Can you work these out from the model? Positions are in its coordinate system, mm. Face numbers are marked on the shaded views. A direction names the side the tool comes from. Give positions to 0.01 mm unless a question says otherwise; leave off trailing zeros. Loops run counter-clockwise (first coordinate to the right, second up) from the corner with the lowest first, then second, coordinate; pieces in that order, holes last. Notation, with made-up numbers: (46.25, 84.5) -> (74.25, 84.5) arc R31 cw to (74.25, 111.5) -> close; hole circle Ø7 at (50.25, -3.75). An arc over 180 degrees is marked (long way). Return JSON: item names as keys, results as strings. Group by question number.
Q1. Suppose I cut it at B-B, the plane z = 5. Please give me the cut outline in (x, y), and give its area (3 significant figures).
Q2. Thinking about a two-plate mould opening in Z: for the marked faces 1, 2, 3 and 4, which applies, pulls with the +Z half, pulls with the -Z half, needs draft (parallel to the pull), parting line crosses it, or undercut?
Q3. Suppose I cut it at D-D, the plane x = -15.5. Please give me the cut outline in (y, z).
Q4. Which directions (+Z, -Z, +X, -X, +Y, -Y) give clear straight access to the entire face, cutting with the end or side of a thin tool? Please do the marked faces 5 and 6.
Q5. Will these pins go through, and if not, where does the flat tip stop? pin 1 (5.5 mm diameter, centred on y = 0, z = 0, fed in from +X); pin 2 (5 mm diameter, centred on y = 2.5, z = -17, fed in from -X); pin 3 (4 mm diameter, centred on y = 5, z = -5, fed in from -X).
Q6. Suppose I cut it at C-C, the plane z = -2. Please give me the cut outline in (x, y).
Q7. I need wall thicknesses on line 1 along Y through (x, z) = (-15.5, 20.95); line 2 along Y through (x, z) = (-8, -21.35); line 3 along Y through (x, z) = (17.25, 5). Which ranges of each line are inside material? Lowest first, please. Write a range as [from, to].
Q8. Suppose I cut it at A-A, the plane x = 10. Please give me the cut outline in (y, z), and give its area (3 significant figures).
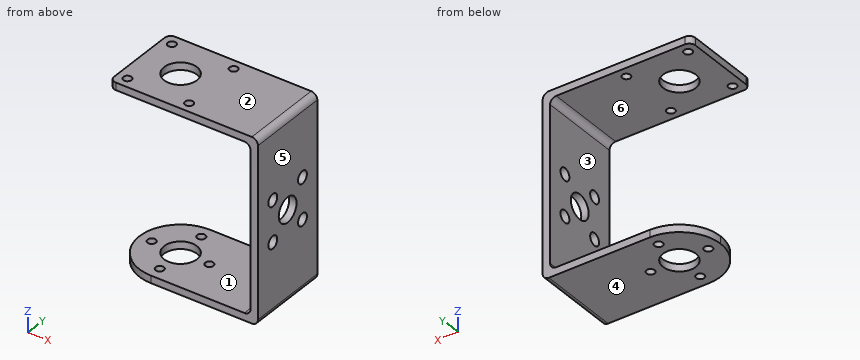
```python
from build123d import *

# Parameters (mm, degrees)
BOSS_EXTRUDE1_DEPTH = 10
FILLET1_R           = 1.5
CUT_EXTRUDE1_DEPTH  = 2
SKETCH4_R           = 4
CUT_EXTRUDE3_DEPTH  = 45.2
SKETCH6_R           = 3
SKETCH6_R_2         = 1.5
CUT_EXTRUDE4_DEPTH  = 2
SKETCH7_R           = 1
CUT_EXTRUDE5_DEPTH  = 2
SKETCH8_R           = 1
CUT_EXTRUDE6_DEPTH  = 2


with BuildPart() as part:
    # Sketch1 → Boss-Extrude1 (new body, symmetric)
    with BuildSketch(Plane(origin=(0, 0, 0), x_dir=(1, 0, 0), z_dir=(0, 1, 0))):
        Polygon((-18, 20.3), (16.2, 20.3), (16.2, -20.3), (-18, -20.3), (-18, -22.1), (18, -22.1), (18, 22.1), (-18, 22.1), align=None)
    extrude(amount=BOSS_EXTRUDE1_DEPTH, both=True)

    # Fillet1
    fillet1_edges = [part.edges().sort_by_distance(p)[0] for p in [
        (18, 0, -22.1),
        (18, 0, 22.1),
        (16.2, 0, 20.3),
        (16.2, 0, -20.3),
        (-18, 10, 21.2),
        (-18, -10, 21.2),
    ]]
    fillet(fillet1_edges, radius=FILLET1_R)

    # Sketch2 → Cut-Extrude1 (cut)
    with BuildSketch(Plane(origin=(0, 0, -22.1), x_dir=(-1, 0, 0), z_dir=(0, 0, -1))):
        with BuildLine():
            Line((18, 10), (8, 10))
            ThreePointArc((8, 10), (15.071067812, 7.071067812), (18, 0))
            Line((18, 0), (18, 10))
        make_face()
        with BuildLine():
            Line((18, -10), (18, 0))
            ThreePointArc((18, 0), (15.071067812, -7.071067812), (8, -10))
            Line((8, -10), (18, -10))
        make_face()
    extrude(amount=-CUT_EXTRUDE1_DEPTH, mode=Mode.SUBTRACT)

    # Sketch4 → Cut-Extrude3 (cut, through all)
    with BuildSketch(Plane.XY.offset(22.1)):
        with Locations((-8, 0)):
            Circle(SKETCH4_R)
    extrude(amount=-CUT_EXTRUDE3_DEPTH, mode=Mode.SUBTRACT)

    # Sketch6 → Cut-Extrude4 (cut)
    with BuildSketch(Plane.ZY.offset(-16.2)):
        Circle(SKETCH6_R)
        with Locations((5, -5)):
            Circle(SKETCH6_R_2)
        with Locations((-5, -5)):
            Circle(SKETCH6_R_2)
        with Locations((-5, 5)):
            Circle(SKETCH6_R_2)
        with Locations((5, 5)):
            Circle(SKETCH6_R_2)
    extrude(amount=-CUT_EXTRUDE4_DEPTH, mode=Mode.SUBTRACT)

    # Sketch7 → Cut-Extrude5 (cut)
    with BuildSketch(Plane.XY.offset(22.1)):
        with Locations((-15.5, -7.5)):
            Circle(SKETCH7_R)
        with Locations((-15.5, 7.5)):
            Circle(SKETCH7_R)
        with Locations((-0.5, 7.5)):
            Circle(SKETCH7_R)
        with Locations((-0.5, -7.5)):
            Circle(SKETCH7_R)
    extrude(amount=-CUT_EXTRUDE5_DEPTH, mode=Mode.SUBTRACT)

    # Sketch8 → Cut-Extrude6 (cut)
    with BuildSketch(Plane(origin=(0, 0, -22.1), x_dir=(-1, 0, 0), z_dir=(0, 0, -1))):
        with Locations((8, -7)):
            Circle(SKETCH8_R)
        with Locations((15, 0)):
            Circle(SKETCH8_R)
        with Locations((8, 7)):
            Circle(SKETCH8_R)
        with Locations((1, 0)):
            Circle(SKETCH8_R)
    extrude(amount=-CUT_EXTRUDE6_DEPTH, mode=Mode.SUBTRACT)


solid = part.part
```
Ans:
{
 "1": {"outline": "(16.2, -10) -> (18, -10) -> (18, -6.5) -> (16.2, -6.5) -> close; (16.2, -3.5) -> (18, -3.5) -> (18, 3.5) -> (16.2, 3.5) -> close; (16.2, 6.5) -> (18, 6.5) -> (18, 10) -> (16.2, 10) -> close", "area": "25.2 mm^2"},
 "2": {"face 1": "undercut", "face 2": "pulls with the +Z half", "face 3": "undercut", "face 4": "pulls with the -Z half"},
 "3": {"outline": "(-10, 20.3) -> (-8.5, 20.3) -> (-8.5, 22.1) -> (-10, 22.1) -> close; (-6.61, -22.1) -> (-0.87, -22.1) -> (-0.87, -20.3) -> (-6.61, -20.3) -> close; (-6.5, 20.3) -> (6.5, 20.3) -> (6.5, 22.1) -> (-6.5, 22.1) -> close; (0.87, -22.1) -> (6.61, -22.1) -> (6.61, -20.3) -> (0.87, -20.3) -> close; (8.5, 20.3) -> (10, 20.3) -> (10, 22.1) -> (8.5, 22.1) -> close"},
 "4": {"face 5": "+Z, -Z, +X, +Y, -Y", "face 6": "-X, +Y, -Y"},
 "5": {"pin 1": "passes through", "pin 2": "stops at x = 16.03", "pin 3": "stops at x = 16.2"},
 "6": {"outline": "(16.2, -10) -> (18, -10) -> (18, -2.24) -> (16.2, -2.24) -> close; (16.2, 2.24) -> (18, 2.24) -> (18, 10) -> (16.2, 10) -> close"},
 "7": {"line 1": "y = [-10, -8.5], [-6.5, 6.5], [8.5, 10]", "line 2": "y = [-10, -8], [-6, -4], [4, 6], [8, 10]", "line 3": "y = [-10, -6.5], [-3.5, 3.5], [6.5, 10]"},
 "8": {"outline": "(-10, -22.1) -> (10, -22.1) -> (10, -20.3) -> (-10, -20.3) -> close; (-10, 20.3) -> (10, 20.3) -> (10, 22.1) -> (-10, 22.1) -> close", "area": "72.0 mm^2"}
}
